Autodesk Inventor part; units mm, degrees
ref_plane "YZ Plane" through (0, 0, 0) normal (1, 0, 0) x (0, 1, 0)
ref_plane "XZ Plane" through (0, 0, 0) normal (0, 1, 0) x (-1, 0, 0)
ref_plane "XY Plane" through (0, 0, 0) normal (0, 0, 1) x (1, 0, 0)
sketch "Sketch1" plane through (0, 0, 0) normal (0, 0, 1) x (1, 0, 0)
  line L0 (0, 0) -> (0, 38.1)
  line L1 (0, 38.1) -> (25.4, 38.1)
  line L2 (25.4, 38.1) -> (25.4, 63.5)
  line L3 (25.4, 63.5) -> (152.4, 63.5)
  line L4 (152.4, 63.5) -> (152.4, 0)
  line L5 (152.4, 0) -> (0, 0)
  dimension "d0" = 152.4
  dimension "d1" = 63.5
  dimension "d2" = 127
  dimension "d3" = 38.1
extrude "Extrusion1" add sketch "Sketch1" along normal blind 12.7
sketch "Sketch2" plane through (0, 0, 12.7) normal (0, 0, 1) x (1, 0, 0)
  line L0 (152.4, 0) -> (152.4, 63.5)
  line L1 (15.24, 12.7) -> (35.56, 12.7) construction
  line L2 (0, 0) -> (152.4, 0) construction
  point P0 (25.4, 22.86)
  dimension "d6" = 127
  dimension "d7" = 10.16
  dimension "d8" = 12.7
  dimension "d9" = 10.16
  dimension "d10" = 10.16
hole "Hole1" at (25.4, 22.86, 12.7) at (15.24, 12.7, 12.7) at (35.56, 12.7, 12.7) direction (0, 0, -1) diameter 6.35 end through all
sketch "Sketch3" plane through (0, 0, 12.7) normal (0, 0, 1) x (1, 0, 0)
  circle A0 centre (68.58, 30.48) radius 22.86 construction
  line L0 (152.4, 0) -> (152.4, 63.5) construction
  line L1 (0, 0) -> (152.4, 0) construction
  line L2 (68.58, 30.48) -> (68.58, 55.3501) construction
  point P0 (68.58, 53.34)
  dimension "d18" = 45.72
  dimension "d19" = 83.82
  dimension "d20" = 30.48
hole "Hole2" at (68.58, 53.34, 12.7) direction (0, 0, -1) diameter 4.7752 end through all
pattern_circular "Circular Pattern1" count 8 over 360 about axis through (68.58, 30.48, 12.7) along (0, 0, 1) of "Hole2"
sketch "Sketch4" plane through (0, 0, 12.7) normal (0, 0, 1) x (1, 0, 0)
  line L0 (152.4, 0) -> (152.4, 63.5) construction
  line L1 (0, 0) -> (152.4, 0)
  point P0 (114.3, 50.8)
  dimension "d32" = 38.1
  dimension "d37" = 50.8
hole "Hole3" at (114.3, 50.8, 12.7) direction (0, 0, -1) diameter 3.175 end through all
pattern_linear "Rectangular Pattern1" count 2 spacing 22.86 along (1, 0, 0) count 3 spacing 20.32 along (0, -1, 0) of "Hole3"
fillet "Fillet1" radius 6.35 4 edges at (25.4, 38.1, 6.35) (0, 38.1, 6.35) (25.4, 63.5, 6.35) (0, 0, 6.35)
properties part number "Plate"
Verification items for the finished model (mm, model axes). A direction names the side the tool comes from. Round coordinates to 2 decimals unless told otherwise and drop trailing zeros. Loops run counter-clockwise (first coordinate to the right, second up) from the corner with the lowest first, then second, coordinate; pieces in that order, holes last. Notation, with made-up numbers: (45, -28) - (70, -28) arc R12 cw to (70, -14) - close; hole circle Ø4 at (14.5, 47). An arc over 180 degrees is marked (long way). Use a Markdown table: item, result. Add a question column.
1. Release check for a two-part mould opening along X. For faces 3 (the face through (1.91, 36.29, 6.44)), 4 (the face through (91, 63.5, 6)), 5 (the face through (115.85, 30.82, 6.26)) record: released by +X, released by -X, zero draft, split by the parting line, or undercut.
2. Section check A-A, the plane x = 91.44. Record the boundary of the cut face in (y, z).
3. Section check B-B, the plane x = 68.58. Record the boundary of the cut face in (y, z), plus the area to 3 significant figures.
4. Section check C-C, the plane y = 14. Record the boundary of the cut face in (x, z).
5. Access from +Z, -Z, +X, -X, +Y, -Y to the whole of each face (thin tool, end or side, straight path). Record for faces 1 (the face through (87.11, 46.96, 6.26)), 2 (the face through (13, 38.1, 6)).
6. Section check D-D, the plane z = 9.5. Give the number of separate pieces and of enclosed holes in the cut face, plus the area to 3 significant figures.
7. Gauge pin test, flat ends, axial feed: pin 1 (3 mm diameter, centred on x = 137.16, y = 30.48, fed in from +Z); pin 2 (6.5 mm diameter, centred on x = 11.5, z = 9, fed in from +Y). Record the tip position at first contact, or that the pin passes through.
8. Thickness scan on probe 1 along Y at (x, z) = (137.16, 3); probe 2 along X at (y, z) = (53.34, 3); probe 3 along X at (y, z) = (22.86, 4.5) (3 decimals). Record the ranges inside material, lowest first. Write a range as [from, to].
Checks:
| question | item | result |
|---|---|---|
| 1 | face 3 | released by -X |
| 1 | face 4 | zero draft |
| 1 | face 5 | undercut |
| 2 | outline | (0, 0) - (28.09, 0) - (28.09, 12.7) - (0, 12.7) - close; (32.87, 0) - (63.5, 0) - (63.5, 12.7) - (32.87, 12.7) - close |
| 3 | outline | (0, 0) - (5.23, 0) - (5.23, 12.7) - (0, 12.7) - close; (10.01, 0) - (50.95, 0) - (50.95, 12.7) - (10.01, 12.7) - close; (55.73, 0) - (63.5, 0) - (63.5, 12.7) - (55.73, 12.7) - close |
| 3 | area | 685 mm^2 |
| 4 | outline | (0, 0) - (12.34, 0) - (12.34, 12.7) - (0, 12.7) - close; (18.14, 0) - (32.66, 0) - (32.66, 12.7) - (18.14, 12.7) - close; (38.46, 0) - (50.05, 0) - (50.05, 12.7) - (38.46, 12.7) - close; (54.78, 0) - (82.38, 0) - (82.38, 12.7) - (54.78, 12.7) - close; (87.11, 0) - (152.4, 0) - (152.4, 12.7) - (87.11, 12.7) - close |
| 5 | face 1 | +Z, -Z |
| 5 | face 2 | +Z, -Z, -X, +Y |
| 6 | separate pieces | 1 |
| 6 | enclosed holes | 17 |
| 6 | area | 8,730 mm^2 |
| 7 | pin 1 | passes through |
| 7 | pin 2 | stops at y = 38.1 |
| 8 | probe 1 | y = [0, 8.57], [11.75, 28.89], [32.07, 49.21], [52.39, 63.5] |
| 8 | probe 2 | x = [25.4, 66.19], [70.97, 152.4] |
| 8 | probe 3 | x = [0, 22.225], [28.575, 152.4] |
